from build123d import *

# Parameters (mm, degrees)
SKETCH1_R           = 55
BOSS_EXTRUDE1_DEPTH = 5
SKETCH2_W           = 15.3
SKETCH2_H           = 15.3
SKETCH2_R           = 1.1
BOSS_EXTRUDE2_DEPTH = 2


with BuildPart() as part:
    # Sketch1 → Boss-Extrude1 (new body)
    with BuildSketch(Plane(origin=(0, 0, 0), x_dir=(0, 0, -1), z_dir=(1, 0, 0))):
        Circle(SKETCH1_R)
        with BuildLine():
            Line((-33.543350277, -37.078884183), (-6.464466094, -10))
            Line((-6.464466094, -10), (6.464466094, -10))
            Line((6.464466094, -10), (33.543350277, -37.078884183))
            ThreePointArc((33.543350277, -37.078884183), (0, -50), (-33.543350277, -37.078884183))
        make_face(mode=Mode.SUBTRACT)
        with BuildLine():
            Line((10, -6.464466094), (10, 6.464466094))
            Line((10, 6.464466094), (37.078884183, 33.543350277))
            ThreePointArc((37.078884183, 33.543350277), (50, 0), (37.078884183, -33.543350277))
            Line((37.078884183, -33.543350277), (10, -6.464466094))
        make_face(mode=Mode.SUBTRACT)
        with BuildLine():
            Line((-37.078884183, 33.543350277), (-10, 6.464466094))
            Line((-10, 6.464466094), (-10, -6.464466094))
            Line((-10, -6.464466094), (-37.078884183, -33.543350277))
            ThreePointArc((-37.078884183, -33.543350277), (-50, 0), (-37.078884183, 33.543350277))
        make_face(mode=Mode.SUBTRACT)
        with BuildLine():
            Line((-0.616796039, -3.445223164), (-4.821572875, -7.65))
            Line((-4.821572875, -7.65), (-7.65, -7.65))
            Line((-7.65, -7.65), (-7.65, -4.821572875))
            Line((-7.65, -4.821572875), (-3.445223164, -0.616796039))
            ThreePointArc((-3.445223164, -0.616796039), (-3.5, 0), (-3.445223164, 0.616796039))
            Line((-3.445223164, 0.616796039), (-7.65, 4.821572875))
            Line((-7.65, 4.821572875), (-7.65, 7.65))
            Line((-7.65, 7.65), (-4.821572875, 7.65))
            Line((-4.821572875, 7.65), (-0.616796039, 3.445223164))
            ThreePointArc((-0.616796039, 3.445223164), (0, 3.5), (0.616796039, 3.445223164))
            Line((0.616796039, 3.445223164), (4.821572875, 7.65))
            Line((4.821572875, 7.65), (7.65, 7.65))
            Line((7.65, 7.65), (7.65, 4.821572875))
            Line((7.65, 4.821572875), (3.445223164, 0.616796039))
            ThreePointArc((3.445223164, 0.616796039), (3.5, 0), (3.445223164, -0.616796039))
            Line((3.445223164, -0.616796039), (7.65, -4.821572875))
            Line((7.65, -4.821572875), (7.65, -7.65))
            Line((7.65, -7.65), (4.821572875, -7.65))
            Line((4.821572875, -7.65), (0.616796039, -3.445223164))
            ThreePointArc((0.616796039, -3.445223164), (0, -3.5), (-0.616796039, -3.445223164))
        make_face(mode=Mode.SUBTRACT)
        with BuildLine():
            Line((6.464466094, 10), (-6.464466094, 10))
            Line((-6.464466094, 10), (-33.543350277, 37.078884183))
            ThreePointArc((-33.543350277, 37.078884183), (0, 50), (33.543350277, 37.078884183))
            Line((33.543350277, 37.078884183), (6.464466094, 10))
        make_face(mode=Mode.SUBTRACT)
    extrude(amount=BOSS_EXTRUDE1_DEPTH)

    # Sketch2 → Boss-Extrude2 (add)
    with BuildSketch(Plane(origin=(5, 0, 0), x_dir=(0, 0, -1), z_dir=(1, 0, 0))):
        Rectangle(SKETCH2_W, SKETCH2_H)
        Circle(SKETCH2_R, mode=Mode.SUBTRACT)
    extrude(amount=-BOSS_EXTRUDE2_DEPTH)


solid = part.part
Work out the finished part from the listing and answer in its coordinate system (mm). A direction names the side the tool comes from. Coordinates: 2 decimals unless noted, no trailing zeros. Loops run counter-clockwise (first coordinate to the right, second up) from the corner with the lowest first, then second, coordinate; pieces in that order, holes last. Notation, with made-up numbers: M 33.25,56.25 L 50.25,56.25 A16 cw 50.25,71.25 Z; hole C 28.5,78 d10. An arc over 180 degrees is marked long. Answer in a Markdown table with one row per item. Add a question column.
1. Find section A-A, the plane z = -14.5. Write down the section's boundary in (x, y).
2. Consider L1, parallel to Y at x = 3.15, z = -33; L2, parallel to Z at x = 0.4, y = 3; L3, parallel to Y at x = 3, z = 22.5. Determine where each line is inside the solid, lowest interval first.
3. Flat-ended cylindrical pins translate along their axes: P1, Ø1.5, axis at x = 1.5, y = 1.5, coming from the -Z side; P2, Ø2.5, axis at x = 1.5, y = 6.5, coming from the +Z side; P3, Ø3, axis at x = 1.5, y = -5.5, coming from the -Z side; P4, Ø5, axis at y = 27.5, z = -35.5, coming from the -X side. Find the tip coordinate at first contact, or state that the pin passes through.
4. A tool of negligible diameter and unlimited length cuts with its end or side. For faces 1 (the flat face through (2, 0, -10)), 2 (the flat face through (5, -4, 0)), 3 (the flat face through (1.48, -2.75, 5.58)), from which of +Z, -Z, +X, -X, +Y, -Y can it reach the whole face along a straight path? Write none if from no direction.
5. Find section C-C, the plane x = 1.4. State how many separate pieces and enclosed holes the cut face has, then the cut area to 3 significant figures.
6. Find section D-D, the plane z = 48. Write down the section's boundary in (x, y).
7. The mould has two halves that part along Z. Classify faces 4 (the cylindrical face through (2.465, -53.692, 11.923)), 5 (the flat face through (2, -10, 0)), 6 (the flat face through (0, -4, 0)): pulls with the +Z half, pulls with the -Z half, needs draft (parallel to the pull), parting line crosses it, or undercut.
8. Find section B-B, the plane y = -21. Write down the section's boundary in (x, z).
Reported:
| question | item | result |
|---|---|---|
| 1 | outline | M 0,-53.05 L 5,-53.05 L 5,-47.85 L 0,-47.85 Z; M 0,-18.04 L 5,-18.04 L 5,-10.96 L 0,-10.96 Z; M 0,10.96 L 5,10.96 L 5,18.04 L 0,18.04 Z; M 0,47.85 L 5,47.85 L 5,53.05 L 0,53.05 Z |
| 2 | L1 | y = -44 to -37.56, -36.54 to -29.46, 29.46 to 36.54, 37.56 to 44 |
| 2 | L2 | z = -54.92 to -49.91, -10 to -5.83, 5.83 to 10, 49.91 to 54.92 |
| 2 | L3 | y = -50.19 to -44.65, -26.04 to -18.96, 18.96 to 26.04, 44.65 to 50.19 |
| 3 | P1 | stops at z = -54.99 |
| 3 | P2 | stops at z = 54.75 |
| 3 | P3 | stops at z = -54.85 |
| 3 | P4 | passes through |
| 4 | face 1 | +X, -X |
| 4 | face 2 | +Z, -Z, +X, +Y, -Y |
| 4 | face 3 | -X |
| 5 | separate pieces | 1 |
| 5 | enclosed holes | 5 |
| 5 | area | 2,650 mm^2 |
| 6 | outline | M 0,-26.85 L 5,-26.85 L 5,-14 L 0,-14 Z; M 0,14 L 5,14 L 5,26.85 L 0,26.85 Z |
| 7 | face 4 | parting line crosses it |
| 7 | face 5 | undercut |
| 7 | face 6 | needs draft |
| 8 | outline | M 0,-50.83 L 5,-50.83 L 5,-45.38 L 0,-45.38 Z; M 0,-24.54 L 5,-24.54 L 5,-17.46 L 0,-17.46 Z; M 0,17.46 L 5,17.46 L 5,24.54 L 0,24.54 Z; M 0,45.38 L 5,45.38 L 5,50.83 L 0,50.83 Z |
